Source: CAD feature listing. Evaluate the final solid. Frame: model axes, mm. Face numbers are marked on the shaded views. Coordinates: 2 decimals unless noted, no trailing zeros. Loops run counter-clockwise (first coordinate to the right, second up) from the corner with the lowest first, then second, coordinate; pieces in that order, holes last.
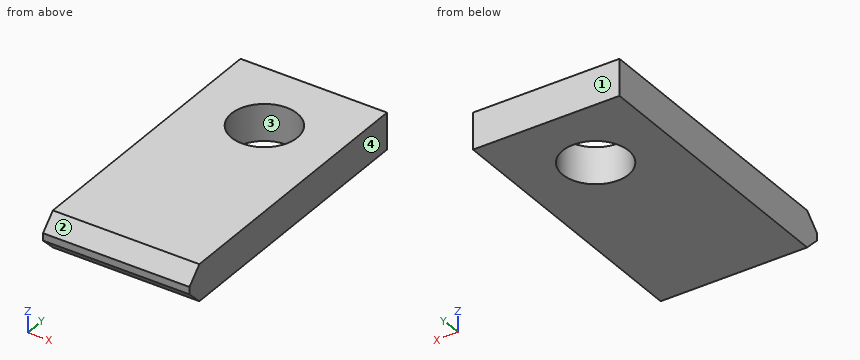
```python
from build123d import *

# Parameters (mm, degrees)
F0_W     = 20
F0_H     = 5
F1_DEPTH = 40
F3_D     = 9
F4_SIZE  = 2


with BuildPart() as f1:
    # F0 (on Front) → F1 (new body)
    with BuildSketch(Plane.XZ):
        Rectangle(F0_W, F0_H)
    extrude(amount=F1_DEPTH)

    # F3 (through all)
    with Locations(Plane.XY.offset(2.5)):
        with Locations((0, -10)):
            Hole(F3_D / 2)

    # F4
    f4_edges = [f1.edges().sort_by_distance(p)[0] for p in [
        (0, -40, 2.5),
        (0, -40, -2.5),
    ]]
    chamfer(f4_edges, length=F4_SIZE)


solid = f1.part
```
Q1. Draft query along Y for the marked faces 1, 2, 3 and 4. Return one class per face: released by +Y, released by -Y, zero draft, split by the parting line, or undercut.
Q2. Section query A-A on y = -10. Return the cut outline in (x, z).
Q3. Section query C-C on z = 1.85. Return the cut outline in (x, y), then the cut area to 3 significant figures.
Q4. Section query B-B on x = 0. Return the cut outline in (y, z), then the cut area to 3 significant figures.
Q5. Material intervals for line 1 along Y through (x, z) = (4, -1.85); line 2 along Y through (x, z) = (-2.25, 1.5); line 3 along X through (y, z) = (-13, 1.65), sorted ascending.
Q6. Section query D-D on x = -7.25. Return the cut outline in (y, z).
Resolved:
1. face 1: released by +Y
1. face 2: released by -Y
1. face 3: undercut
1. face 4: zero draft
2. outline: (-10, -2.5) - (-4.5, -2.5) - (-4.5, 2.5) - (-10, 2.5) - close; (4.5, -2.5) - (10, -2.5) - (10, 2.5) - (4.5, 2.5) - close
3. outline: (-10, -38.65) - (10, -38.65) - (10, 0) - (-10, 0) - close; hole circle Ø9 at (0, -10)
3. area: 709 mm2
4. outline: (-40, -0.5) - (-38, -2.5) - (-14.5, -2.5) - (-14.5, 2.5) - (-38, 2.5) - (-40, 0.5) - close; (-5.5, -2.5) - (0, -2.5) - (0, 2.5) - (-5.5, 2.5) - close
4. area: 151 mm2
5. line 1: y = -38.65 to -12.06, -7.94 to 0
5. line 2: y = -39 to -13.9, -6.1 to 0
5. line 3: x = -10 to -3.35, 3.35 to 10
6. outline: (-40, -0.5) - (-38, -2.5) - (0, -2.5) - (0, 2.5) - (-38, 2.5) - (-40, 0.5) - close
